Could you check a few things on this drawing? It's one solid part, dimensions in mm from its lowest x, y, z. Round coordinates to 2 decimals unless told otherwise and drop trailing zeros. Write each loop counter-clockwise with the first axis right and the second up, starting at its lowest first coordinate (ties: lowest second). Pieces come first, ordered by that corner, then holes. Notation, with made-up numbers: (62.25, 80) - (69.25, 80) arc R25 cw to (69.25, 93) - close; hole circle Ø6 at (-22, 32). An arc over 180 degrees is marked (long way). Use one line per item in the form item = value. Start each with the question number.
1. I want a section at B-B, the plane x = 93.5. List the corners of the cut face in (y, z) for me.
2. If I drill on line 1 along Y through (x, z) = (7.5, 2.55), over which ranges is the centre line in solid material (lowest first)?
3. I want a section at A-A, the plane z = 2.5. List the corners of the cut face in (x, y) for me.
4. Will these pins go through, and if not, where does the flat tip stop? pin 1 (0.9 mm diameter, centred on y = 1, z = 2, fed in from -X); pin 2 (0.9 mm diameter, centred on x = 91.5, z = 2, fed in from +Y); pin 3 (1.5 mm diameter, centred on y = 2, z = 2, fed in from +X).
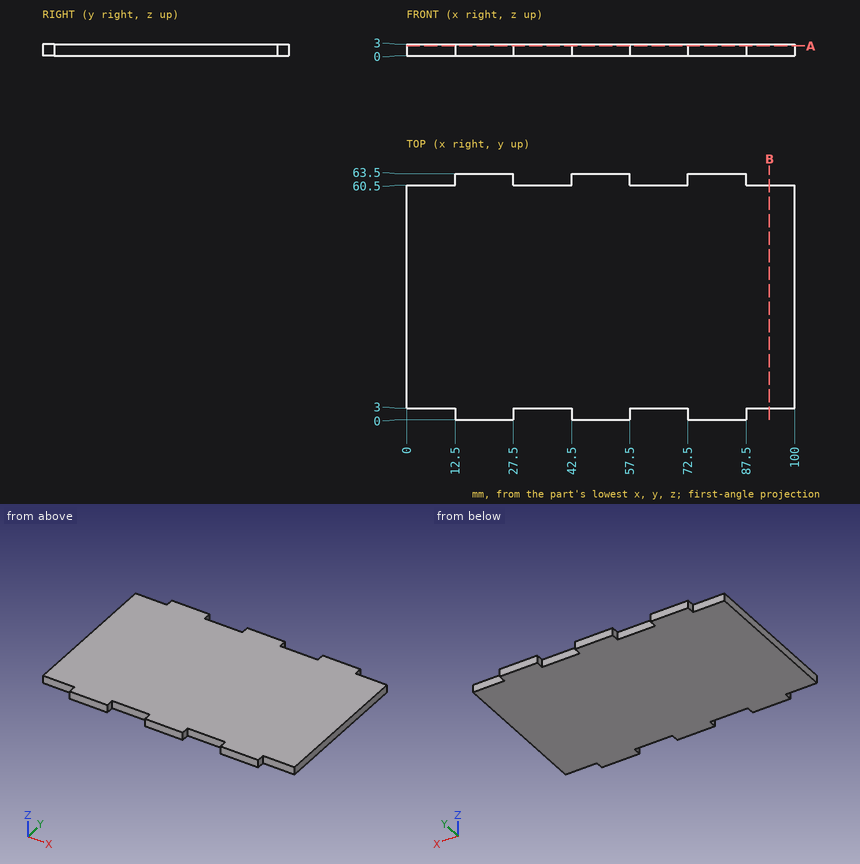
Model answer:
q1.outline = (3, 0) - (60.5, 0) - (60.5, 3) - (3, 3) - close
q2.line_1 = 3 to 60.5
q3.outline = (0, 3) - (12.5, 3) - (12.5, 0) - (27.5, 0) - (27.5, 3) - (42.5, 3) - (42.5, 0) - (57.5, 0) - (57.5, 3) - (72.5, 3) - (72.5, 0) - (87.5, 0) - (87.5, 3) - (100, 3) - (100, 60.5) - (87.5, 60.5) - (87.5, 63.5) - (72.5, 63.5) - (72.5, 60.5) - (57.5, 60.5) - (57.5, 63.5) - (42.5, 63.5) - (42.5, 60.5) - (27.5, 60.5) - (27.5, 63.5) - (12.5, 63.5) - (12.5, 60.5) - (0, 60.5) - close
q4.pin_1 = 12.5
q4.pin_2 = 60.5
q4.pin_3 = 87.5
